```python
from build123d import *

# Parameters (mm, degrees)
CUT_EXTRUDE1_START = -10
SKETCH2_W          = 22.11
SKETCH2_H          = 3.04
CUT_EXTRUDE1_DEPTH = 57.908847779
CIRPATTERN1_COUNT  = 4
FILLET1_R          = 1.5


with BuildPart() as part:
    # Sketch1 → Revolve1 (revolve)
    with BuildSketch(Plane.XY):
        with BuildLine():
            Line((0, 0), (0, 21))
            ThreePointArc((0, 21), (11.593101397, 23.173836988), (21.611108255, 29.4))
            Line((21.611108255, 29.4), (25.846469778, 29.4))
            ThreePointArc((25.846469778, 29.4), (16.827157621, 22.310477905), (6, 18.518120701))
            Line((6, 18.518120701), (6, 0))
            Line((6, 0), (0, 0))
        make_face()
    revolve(axis=Axis((0, 0, 0), (0, 1, 0)))

    # Sketch2 → Cut-Extrude1 (cut)
    with BuildSketch(Plane.XY.offset(CUT_EXTRUDE1_START)):
        with Locations((0, 27.88)):
            Rectangle(SKETCH2_W, SKETCH2_H)
    cut_extrude1 = extrude(amount=CUT_EXTRUDE1_DEPTH, mode=Mode.SUBTRACT)

    # CirPattern1: Cut-Extrude1 ×4 about axis
    cirpattern1_axis = Axis((0, 0, 0), (0, 1, 0))
    for i in range(1, CIRPATTERN1_COUNT):
        add(cut_extrude1.rotate(cirpattern1_axis, i * 360 / CIRPATTERN1_COUNT), mode=Mode.SUBTRACT)

    # Fillet1
    fillet1_edges = [part.edges().sort_by_distance(p)[0] for p in [
        (-6, 18.518120701, 0),
    ]]
    fillet(fillet1_edges, radius=FILLET1_R)


solid = part.part
```
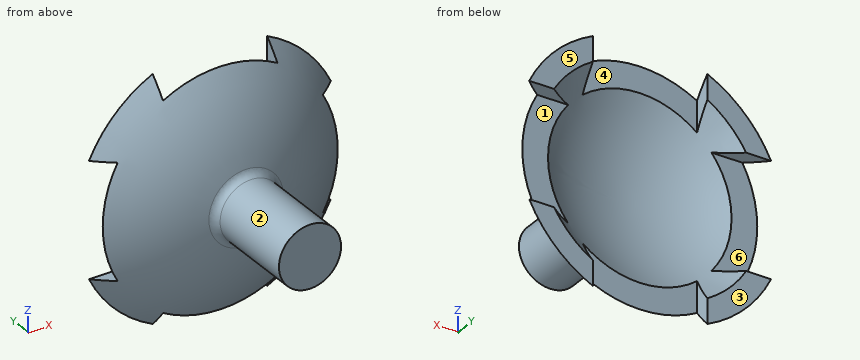
CAD build for the part. Positions are in the model's coordinates, mm. Face numbers are marked on the shaded views. A direction names the side the tool comes from. Round coordinates to 2 decimals unless told otherwise and drop trailing zeros. Order: outer loops, then holes, each group sorted by start corner. A loop starts at its lowest first (then second) coordinate and runs counter-clockwise, first axis right, second up.
Q1. Two-plate mould, pull along Z, no slides. Class the marked faces 1, 2 and 3: pulls with the +Z half, pulls with the -Z half, needs draft (parallel to the pull), parting line crosses it, or undercut.
Q2. Slice it at B-B (y = 24.5). Write the cut outline in (x, z).
Q3. Wall check: L1, parallel to Z at x = 3, y = 24.5; L2, parallel to Z at x = 21, y = 28 (3 decimals); L3, parallel to Y at x = 2, z = -18.5. Give the ranges that are in metal, low to high.
Q4. Slice it at D-D (z = 10). Write the cut outline in (x, y), and give its area (3 significant figures).
Q5. Drop flat-ended pins along their axis: pin 1 (2.5 mm diameter, centred on y = 28, z = -18, fed in from +X); pin 2 (10 mm diameter, centred on y = 22, z = -14, fed in from -X); pin 3 (3.5 mm diameter, centred on x = -16.5, y = 28, fed in from -Z). Give the stop position or say it passes through.
Q6. Slice it at C-C (y = 3). Write the cut outline in (x, z), and give its area (3 significant figures).
Q7. Slice it at A-A (x = 15). Write the cut outline in (y, z) (3 decimals), and give its area (3 significant figures).
Q8. Which spindle directions (+Z, -Z, +X, -X, +Y, -Y) get a long thin tool onto all of the face, cutting with end or side? Do the marked faces 4, 5 and 6. Say none if no direction does.
Results below:
1. face 1: undercut
1. face 2: parting line crosses it
1. face 3: needs draft
2. outline: circle Ø40.63 at (0, 0); hole circle Ø29.1 at (0, 0)
3. L1: z = -20.09 to -14.24, 14.24 to 20.09
3. L2: z = -12.61 to -11.055, 11.055 to 12.61
3. L3: y = 23.36 to 26.36
4. outline: (-20.38, 26.36) arc R33.54 ccw to (20.38, 26.36) - (14.64, 26.36) arc R30.4 cw to (-14.64, 26.36) - close
4. area: 117 mm2
5. pin 1: stops at x = 18.75
5. pin 2: stops at x = -19.57
5. pin 3: stops at z = -20.72
6. outline: circle Ø12 at (0, 0)
6. area: 113 mm2
7. outline: (26.36, -11.055) - (26.36, -9.45) arc R28.267 cw to (26.36, 9.45) - (26.36, 11.055) - (26.985, 11.055) arc R28.267 cw to (29.4, 15.558) - (29.4, 21.049) arc R31.623 ccw to (29.4, -21.049) - (29.4, -15.558) arc R28.267 cw to (26.985, -11.055) - close
7. area: 132 mm2
8. face 4: +Z, -Z, +Y
8. face 5: +Z, -Z, +X, -X, +Y
8. face 6: +X, -X, +Y
